Could you check a few things on this model? Use its own coordinates, in mm. Give positions to 0.01 mm unless a question says otherwise; leave off trailing zeros. Write each loop counter-clockwise with the first axis right and the second up, starting at its lowest first coordinate (ties: lowest second). Pieces come first, ordered by that corner, then holes. Notation, with made-up numbers: (-13.5, 81.5) - (9.5, 81.5) arc R11 ccw to (9.5, 92.5) - close; hole circle Ø3 at (-35.5, 31.25). An arc over 180 degrees is marked (long way). Answer as CSV lines item,"result". Start each with the question number.
Q1. Will these pins go through, and if not, where does the flat tip stop? pin 1 Ø3.5 at (x, y) = (0, 3.5) entering from -Z; pin 2 Ø4 at (x, y) = (-25, 3.7) entering from -Z.
Q2. If I drill on line 1 along X through (y, z) = (3.7, -0.05); line 2 along X through (y, z) = (3.75, 7.5); line 3 along Y through (x, z) = (0, -0.1), over which ranges is the centre line in solid material (lowest first)?
Q3. Imagine slicing it at B-B on z = 2. List the corners of the cut face in (x, y) for me.
Q4. Imagine slicing it at A-A on x = 25. List the corners of the cut face in (y, z) for me, and give its area (3 significant figures).
```python
from build123d import *

# Parameters (mm, degrees)
SKETCH_W            = 60
SKETCH_H            = 15
PAD_DEPTH           = 8.51
SKETCH001_R         = 1.6
POCKET_DEPTH        = 8.511
SKETCH002_R         = 2.3
POCKET001_DEPTH     = 5.1
POCKET001_FACE1_W   = 60
POCKET001_FACE1_H   = 8.51
PAD001_DEPTH        = 2.3
PAD001_FACE1_W      = 60
PAD001_FACE1_H      = 8.51
POCKET002_DEPTH     = 5.3
POCKET002_FACE2_W   = 12
POCKET002_FACE2_H   = 60
POCKET002_FACE2_R   = 1.6
POCKET002_FACE2_R_2 = 2.3
PAD002_DEPTH        = 0.15
PAD002_FACE10_W     = 12
PAD002_FACE10_H     = 8.66
PAD003_DEPTH        = 70
PAD003_FACE3_W      = 12
PAD003_FACE3_H      = 8.66
PAD004_DEPTH        = 70


with BuildPart() as part:
    # Sketch → Pad (new body)
    with BuildSketch(Plane.XY):
        with Locations((0, 7.5)):
            Rectangle(SKETCH_W, SKETCH_H)
    extrude(amount=PAD_DEPTH)

    # Sketch001 (on Face6 of Pad) → Pocket (cut, through all)
    with BuildSketch(Plane.XY.offset(8.51)):
        with Locations((0, 3.5)):
            Circle(SKETCH001_R)
    extrude(amount=-POCKET_DEPTH, mode=Mode.SUBTRACT)

    # Sketch002 (on Face4 of Pocket) → Pocket001 (cut)
    with BuildSketch(Plane(origin=(0, 0, 0), x_dir=(1, 0, 0), z_dir=(0, 0, -1))):
        with Locations((-25, -3.7)):
            Circle(SKETCH002_R)
        with Locations((25, -3.7)):
            Circle(SKETCH002_R)
    extrude(amount=-POCKET001_DEPTH, mode=Mode.SUBTRACT)

    # Pocket001 Face1 → Pad001 (add)
    with BuildSketch(Plane(origin=(0, 0, 4.255), x_dir=(-1, 0, 0), z_dir=(0, -1, 0))):
        Rectangle(POCKET001_FACE1_W, POCKET001_FACE1_H)
    extrude(amount=PAD001_DEPTH)

    # Pad001 Face1 → Pocket002 (cut)
    with BuildSketch(Plane(origin=(0, 15, 4.255), x_dir=(1, 0, 0), z_dir=(0, 1, 0))):
        Rectangle(PAD001_FACE1_W, PAD001_FACE1_H)
    extrude(amount=-POCKET002_DEPTH, mode=Mode.SUBTRACT)

    # Pocket002 Face2 → Pad002 (add)
    with BuildSketch(Plane(origin=(0, 3.70237, 0), x_dir=(0, -1, 0), z_dir=(0, 0, -1))):
        with Locations((0.00237, 0)):
            Rectangle(POCKET002_FACE2_W, POCKET002_FACE2_H)
        with Locations((0.20237, 0)):
            Circle(POCKET002_FACE2_R, mode=Mode.SUBTRACT)
        with Locations((0.00237, -25)):
            Circle(POCKET002_FACE2_R_2, mode=Mode.SUBTRACT)
        with Locations((0.00237, 25)):
            Circle(POCKET002_FACE2_R_2, mode=Mode.SUBTRACT)
    extrude(amount=PAD002_DEPTH)

    # Pad002 Face10 → Pad003 (add)
    with BuildSketch(Plane(origin=(-30, 3.7, 4.18), x_dir=(0, 1, 0), z_dir=(-1, 0, 0))):
        Rectangle(PAD002_FACE10_W, PAD002_FACE10_H)
    extrude(amount=PAD003_DEPTH)

    # Pad003 Face3 → Pad004 (add)
    with BuildSketch(Plane(origin=(30, 3.7, 4.18), x_dir=(0, -1, 0), z_dir=(1, 0, 0))):
        Rectangle(PAD003_FACE3_W, PAD003_FACE3_H)
    extrude(amount=PAD004_DEPTH)


solid = part.part
```
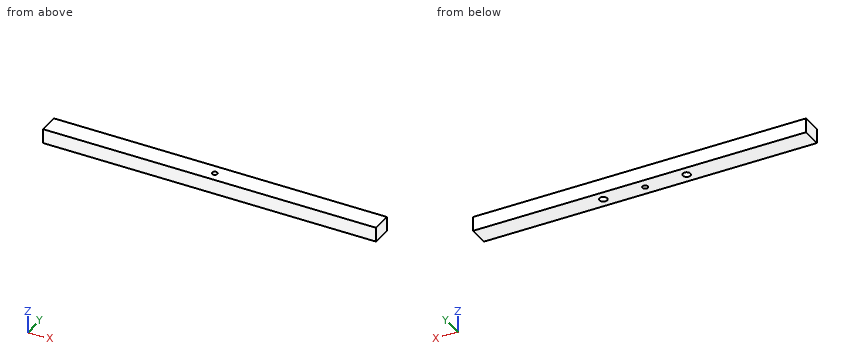
Conclusion:
1,pin 1,"z = -0.15"
1,pin 2,"z = 5.1"
2,line 1,"-100 to -27.3, -22.7 to -1.59, 1.59 to 22.7, 27.3 to 100"
2,line 2,"-100 to -1.58, 1.58 to 100"
2,line 3,"-2.3 to 1.9, 5.1 to 9.7"
3,outline,"(-100, -2.3) - (100, -2.3) - (100, 9.7) - (-100, 9.7) - close; hole circle Ø4.6 at (-25, 3.7); hole circle Ø3.2 at (0, 3.5); hole circle Ø4.6 at (25, 3.7)"
4,outline,"(-2.3, -0.15) - (1.4, -0.15) - (1.4, 5.1) - (6, 5.1) - (6, -0.15) - (9.7, -0.15) - (9.7, 8.51) - (-2.3, 8.51) - close"
4,area,"79.8 mm^2"
